The listing builds one solid part. Answer for the finished solid, in the listing's coordinates (mm). A direction names the side the tool comes from. Round coordinates to 2 decimals unless told otherwise and drop trailing zeros. Order: outer loops, then holes, each group sorted by start corner. A loop starts at its lowest first (then second) coordinate and runs counter-clockwise, first axis right, second up. Notation, with made-up numbers: (-24, -13.75) -> (32, -13.75) arc R9 cw to (32, 3.25) -> close; hole circle Ø9 at (8, -27.75). An arc over 180 degrees is marked (long way). Answer in a Markdown table with one row per item. Add a question column.
```python
from build123d import *
from build123d.topology import SkipClean

# Parameters (mm, degrees)
SKETCH2_W             = 8
SKETCH2_H             = 3.5
BOSS_EXTRUDE2_DEPTH   = 35
BOSS_EXTRUDE2_2_DEPTH = 35
SKETCH2_3_W           = 8
SKETCH2_3_H           = 29.15
BOSS_EXTRUDE3_DEPTH   = 2
SKETCH7_W             = 4
SKETCH7_H             = 36.15
BOSS_EXTRUDE4_DEPTH   = 15
CUT_EXTRUDE5_REACH    = 51.739
SKETCH8_R             = 1.1
SKETCH8_W             = 12
SKETCH8_H             = 23
CUT_EXTRUDE6_DEPTH    = 1.4
SKETCH10_R            = 3.45
CUT_EXTRUDE7_DEPTH    = 52.060667156


with BuildPart() as part:
    # Sketch2 → Boss-Extrude2 (new body)
    with BuildSketch(Plane.XY):
        with Locations((-4.681545395, -0.713506952)):
            Rectangle(SKETCH2_W, SKETCH2_H)
    extrude(amount=BOSS_EXTRUDE2_DEPTH)

    # Sketch2_3 → Boss-Extrude3 (add)
    with BuildSketch(Plane.XY):
        with Locations((-4.681545395, -17.038506952)):
            Rectangle(SKETCH2_3_W, SKETCH2_3_H)
    extrude(amount=BOSS_EXTRUDE3_DEPTH)



with BuildPart() as body_2:
    # Sketch2 → Boss-Extrude2 2 (new body)
    with BuildSketch(Plane.XY):
        with Locations((-4.681545395, -33.363506952)):
            Rectangle(SKETCH2_W, SKETCH2_H)
    extrude(amount=BOSS_EXTRUDE2_2_DEPTH)


with BuildPart() as part_1:
    add(part.part)

    add(body_2.part)  # Boss-Extrude4 merges body 2
    # Sketch7 → Boss-Extrude4 (add)
    with BuildSketch(Plane(origin=(0, 0, 0), x_dir=(-1, 0, 0), z_dir=(0, 0, -1))):
        with Locations((6.681545395, -17.038506952)):
            Rectangle(SKETCH7_W, SKETCH7_H)
    extrude(amount=BOSS_EXTRUDE4_DEPTH)

    # Sketch8 → Cut-Extrude5 (cut, up to next)
    with BuildSketch(Plane(origin=(-4.681545395, 0, 0), x_dir=(0, 0, -1), z_dir=(1, 0, 0)), mode=Mode.PRIVATE) as cut_extrude5_sk1:
        with Locations((7.5, -2.888506952)):
            Circle(SKETCH8_R)
    cut_extrude5_tool1 = extrude(cut_extrude5_sk1.sketch, amount=-CUT_EXTRUDE5_REACH, mode=Mode.PRIVATE) & part_1.part
    # Sketch8 → Cut-Extrude5 (cut, up to next)
    with BuildSketch(Plane(origin=(-4.681545395, 0, 0), x_dir=(0, 0, -1), z_dir=(1, 0, 0)), mode=Mode.PRIVATE) as cut_extrude5_sk2:
        with Locations((7.5, -31.188506952)):
            Circle(SKETCH8_R)
    cut_extrude5_tool2 = extrude(cut_extrude5_sk2.sketch, amount=-CUT_EXTRUDE5_REACH, mode=Mode.PRIVATE) & part_1.part
    # Sketch8 → Cut-Extrude5 (cut, up to next)
    with BuildSketch(Plane(origin=(-4.681545395, 0, 0), x_dir=(0, 0, -1), z_dir=(1, 0, 0)), mode=Mode.PRIVATE) as cut_extrude5_sk3:
        with Locations((7.5, -17.038506952)):
            Rectangle(SKETCH8_W, SKETCH8_H)
    cut_extrude5_tool3 = extrude(cut_extrude5_sk3.sketch, amount=-CUT_EXTRUDE5_REACH, mode=Mode.PRIVATE) & part_1.part
    add(cut_extrude5_tool1.solids().sort_by_distance((-4.681545, -2.888507, -7.5))[0], mode=Mode.SUBTRACT)
    add(cut_extrude5_tool2.solids().sort_by_distance((-4.681545, -31.188507, -7.5))[0], mode=Mode.SUBTRACT)
    add(cut_extrude5_tool3.solids().sort_by_distance((-4.681545, -17.038507, -7.5))[0], mode=Mode.SUBTRACT)

    # Sketch9 → Cut-Extrude6 (cut)
    with BuildSketch(Plane(origin=(0, 1.036493048, 0), x_dir=(1, 0, 0), z_dir=(0, 1, 0))):
        with BuildLine():
            Line((-2.684524514, -15.840878033), (-2.031545395, -27.790927797))
            ThreePointArc((-2.031545395, -27.790927797), (-4.681545395, -33.45), (-7.331545395, -27.790927797))
            Line((-7.331545395, -27.790927797), (-6.678566275, -15.840878033))
            ThreePointArc((-6.678566275, -15.840878033), (-4.681545395, -13.95), (-2.684524514, -15.840878033))
        make_face()
    extrude(amount=-CUT_EXTRUDE6_DEPTH, mode=Mode.SUBTRACT)

    # Sketch10 → Cut-Extrude7 (cut, through all)
    with SkipClean():  # the faces are left unmerged after this step: merging them gives an invalid solid
        with BuildSketch(Plane(origin=(0, 1.036493048, 0), x_dir=(1, 0, 0), z_dir=(0, 1, 0))):
            with Locations(Location((-4.681545395, -30, 0), (0, 0, 180))):
                Circle(SKETCH10_R)
        extrude(amount=-CUT_EXTRUDE7_DEPTH, mode=Mode.SUBTRACT)


solid = part_1.part
```
Item 1: The part is cut by section A-A, the plane y = -10.5. Give the vertices of the cut face in (x, z).
Item 2: Find the intervals of material crossed by probe 1 along Y at (x, z) = (-6.95, -7.5); probe 2 along Z at (x, y) = (-5.25, -21.5); probe 3 along Y at (x, z) = (-5.25, 4.5), in increasing order. Write a range as [from, to].
Item 3: The part is cut by section B-B, the plane z = -4.5. Give the vertices of the cut face in (x, y), and give its area (3 significant figures).
Item 4: The part is cut by section D-D, the plane x = -3.75. Give the vertices of the cut face in (y, z).
Item 5: A tool of negligible diameter and unlimited length cuts with its end or side. For faces 5 (the face through (-3, -17, 0)), 6 (the face through (-7.01, 0.35, 21.9)), 7 (the face through (-5, -31.614, 15)), 8 (the face through (-7, -17, -1.5)), from which of +Z, -Z, +X, -X, +Y, -Y can it reach the whole face along a straight path? Write none if from no direction.
Item 6: Flat-ended cylindrical pins translate along their axes: P1, Ø2, axis at x = -7, y = -18.5, coming from the +Z side; P2, Ø2, axis at x = -3.5, y = -12.5, coming from the -Z side. Find the tip coordinate at first contact, or state that the pin passes through.
Item 7: For a pull along Z with two mould halves and no side action, classify faces 1 (the face through (-7, -17, -15)), 2 (the face through (-5, -17, 2)), 3 (the face through (-6.654, -3.31, -8.516)), 4 (the face through (-5, -2.464, 15)) as released by +Z, released by -Z, zero draft, split by the parting line, or undercut.
Item 8: The part is cut by section C-C, the plane x = -6. Give the vertices of the cut face in (y, z).
Resolved:
| question | item | result |
|---|---|---|
| 1 | outline | (-8.68, -15) -> (-4.68, -15) -> (-4.68, -13.5) -> (-8.68, -13.5) -> close; (-8.68, -1.5) -> (-4.68, -1.5) -> (-4.68, 0) -> (-0.68, 0) -> (-0.68, 2) -> (-8.68, 2) -> close |
| 2 | probe 1 | [-35.11, -32.29], [-30.09, -28.54], [-5.54, -3.99], [-1.79, 1.04] |
| 2 | probe 2 | [-15, -13.5], [-1.5, 2] |
| 2 | probe 3 | [-35.11, -31.61], [-2.46, 1.04] |
| 3 | outline | (-8.68, -35.11) -> (-4.68, -35.11) -> (-4.68, -28.54) -> (-8.68, -28.54) -> close; (-8.68, -5.54) -> (-4.68, -5.54) -> (-4.68, 1.04) -> (-8.68, 1.04) -> close |
| 3 | area | 52.6 mm2 |
| 4 | outline | (-35.11, 0) -> (1.04, 0) -> (1.04, 14.18) -> (-0.36, 14.18) -> (-0.36, 26.68) -> (-2.46, 26.68) -> (-2.46, 2) -> (-31.61, 2) -> (-31.61, 26.68) -> (-35.11, 26.68) -> close; (-35.11, 33.32) -> (-31.61, 33.32) -> (-31.61, 35) -> (-35.11, 35) -> close; (-2.46, 33.32) -> (1.04, 33.32) -> (1.04, 35) -> (-2.46, 35) -> close |
| 5 | face 5 | -Z, +X, +Y, -Y |
| 5 | face 6 | +Y |
| 5 | face 7 | +Z, +X, -X |
| 5 | face 8 | +X, -X |
| 6 | P1 | z = 2 |
| 6 | P2 | z = 0 |
| 7 | face 1 | released by -Z |
| 7 | face 2 | released by +Z |
| 7 | face 3 | undercut |
| 7 | face 4 | zero draft |
| 8 | outline | (-35.11, -15) -> (1.04, -15) -> (1.04, 14.45) -> (-0.36, 14.45) -> (-0.36, 26.81) -> (-2.46, 26.81) -> (-2.46, 2) -> (-31.61, 2) -> (-31.61, 26.81) -> (-35.11, 26.81) -> close; (-35.11, 33.19) -> (-31.61, 33.19) -> (-31.61, 35) -> (-35.11, 35) -> close; (-2.46, 33.19) -> (1.04, 33.19) -> (1.04, 35) -> (-2.46, 35) -> close; hole circle Ø2.2 at (-31.19, -7.5); hole (-28.54, -13.5) -> (-5.54, -13.5) -> (-5.54, -1.5) -> (-28.54, -1.5) -> close; hole circle Ø2.2 at (-2.89, -7.5) |
